Input: dimensioned drawing with shaded views. Units: mm. Origin: part minimum x, y, z. Coordinates: 2 decimals unless noted, no trailing zeros. Order: outer loops, then holes, each group sorted by start corner. A loop starts at its lowest first (then second) coordinate and runs counter-clockwise, first axis right, second up. Notation, with made-up numbers: (-8, -25) -> (1, -25) arc R28 cw to (1, 0) -> close; hole circle Ø7 at (86, -5.5). An arc over 180 degrees is marked (long way). Answer as CSV lines item,"result".
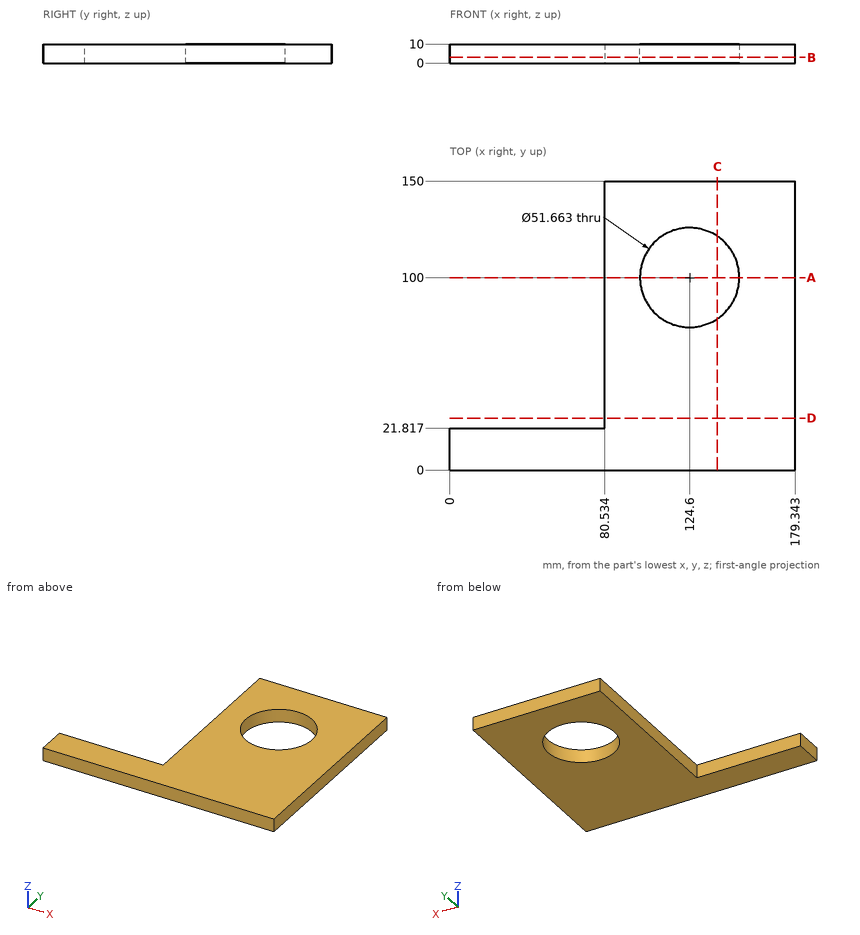
1. Cut plane A-A (y = 100). Return the cut outline in (x, z).
Findings:
outline,"(80.53, 0) -> (98.77, 0) -> (98.77, 10) -> (80.53, 10) -> close; (150.43, 0) -> (179.34, 0) -> (179.34, 10) -> (150.43, 10) -> close"
2. Contact query for a flat-ended pin moving along its axis: pin 1 (1.5 mm diameter, centred on y = 54, z = 2.5, fed in from -X). Output: stop coordinate, or through.
Findings:
pin 1,"stops at x = 80.53"
3. Cut plane D-D (y = 27). Return the cut outline in (x, z), plus the area to 3 significant figures.
Findings:
outline,"(80.53, 0) -> (179.34, 0) -> (179.34, 10) -> (80.53, 10) -> close"
area,"988 mm2"
4. Ray query, line 1 along X through (y, z) = (47, 4); line 2 along Y through (x, z) = (137, 9.25); line 3 along X through (y, z) = (94, 8.75) (1 decimal). Return the intervals inside material, ascending.
Findings:
line 1,"x = 80.53 to 179.34"
line 2,"y = 0 to 77.34, 122.66 to 150"
line 3,"x = 80.5 to 99.5, 149.7 to 179.3"
5. Cut plane B-B (z = 3). Return the cut outline in (x, y).
Findings:
outline,"(0, 0) -> (179.34, 0) -> (179.34, 150) -> (80.53, 150) -> (80.53, 21.82) -> (0, 21.82) -> close; hole circle Ø51.66 at (124.6, 100)"
6. Cut plane C-C (x = 139). Return the cut outline in (y, z) (1 decimal), plus the area to 3 significant figures.
Findings:
outline,"(0, 0) -> (78.6, 0) -> (78.6, 10) -> (0, 10) -> close; (121.4, 0) -> (150, 0) -> (150, 10) -> (121.4, 10) -> close"
area,"1,070 mm2"
